The model under review builds one solid part; all positions refer to its coordinate system, in mm. Face numbers are marked on the shaded views. A direction names the side the tool comes from. Round coordinates to 2 decimals unless told otherwise and drop trailing zeros. Order: outer loops, then holes, each group sorted by start corner. A loop starts at its lowest first (then second) coordinate and runs counter-clockwise, first axis right, second up. Notation, with made-up numbers: M 27,17.25 L 32,17.25 A23 cw 32,38.25 Z; hole C 16,-17 d11. An arc over 180 degrees is marked long. One line per item, written item: value. Start each with the question number.
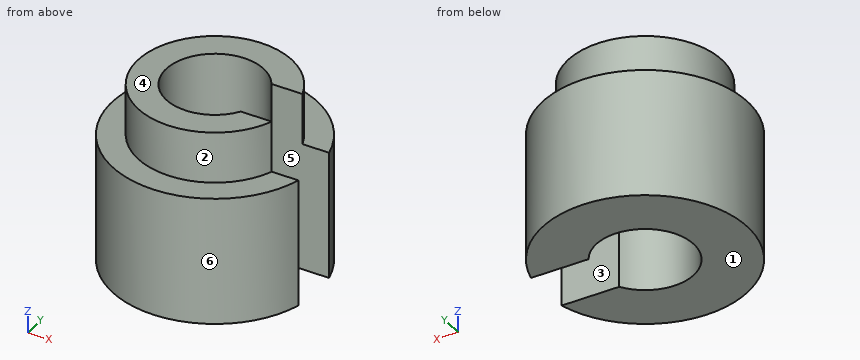
from build123d import *

# Parameters (mm, degrees)
SKETCH_1_R          = 4
EXTRUDE_1_DEPTH     = 5
SKETCH_2_R          = 3
EXTRUDE_2_DEPTH     = 2
SKETCH_3_R          = 1.9
CUT_EXTRUDE_1_DEPTH = 10
CUT_EXTRUDE_2_DEPTH = 1


with BuildPart() as part:
    # 草图1 → 凸台-拉伸1 (new body)
    with BuildSketch(Plane.XY):
        Circle(SKETCH_1_R)
    extrude(amount=EXTRUDE_1_DEPTH)

    # 草图2 → 凸台-拉伸2 (add)
    with BuildSketch(Plane.XY.offset(5)):
        Circle(SKETCH_2_R)
    extrude(amount=EXTRUDE_2_DEPTH)

    # 草图3 → 切除-拉伸1 (cut, through all)
    with BuildSketch(Plane.XY.offset(7)):
        Circle(SKETCH_3_R)
    extrude(amount=-CUT_EXTRUDE_1_DEPTH, mode=Mode.SUBTRACT)

    # 草图4 → 切除-拉伸2 (cut, symmetric)
    with BuildSketch(Plane(origin=(0, 0, 0), x_dir=(1, 0, 0), z_dir=(0, 1, 0))):
        Polygon((0, 0), (4, 0), (4, -5), (3, -5), (3, -7), (0, -7), align=None)
    extrude(amount=CUT_EXTRUDE_2_DEPTH, both=True, mode=Mode.SUBTRACT)


solid = part.part
Item 1: Consider section D-D, the plane z = 6. Give the boundary of the cut face in (x, y).
Item 2: Consider section B-B, the plane y = -1.5. Give the boundary of the cut face in (x, z).
Item 3: Machinability: for the marked faces 1, 2 and 3, which of the approach directions +Z, -Z, +X, -X, +Y, -Y give a long, thin tool a straight path to every point of the face, cutting with its end or side? Answer none if there is none.
Item 4: Consider section C-C, the plane y = 0. Give the boundary of the cut face in (x, z), then the cut area to 3 significant figures.
Item 5: Wall thickness on L1, parallel to Z at x = -1.75, y = -2.75; L2, parallel to Y at x = 2, z = 1.25; L3, parallel to X at y = 0, z = 2.75: over which ranges is each line inside the solid? List them lowest first.
Item 6: Consider section A-A, the plane x = 0. Give the boundary of the cut face in (y, z).
Item 7: The part is to be moulded in two halves that separate along Y. For the marked faces 4, 5 and 6, say which applies: pulls with the +Y half, pulls with the -Y half, needs draft (parallel to the pull), parting line crosses it, or undercut.
Item 8: Clearance check with flat-ended pins moving along their axes: P1, Ø1.5, axis at x = -2.5, z = 4, coming from the +Y side; P2, Ø0.7, axis at x = 2.5, z = 2.5, coming from the -Y side; P3, Ø1.1, axis at x = 3.5, z = 4.5, coming from the +Y side. State where each tip first meets the part, or that it passes through.
Computed:
1. outline: M 1.62,-1 A1.9 cw long 1.62,1 L 2.83,1 A3 ccw long 2.83,-1 Z
2. outline: M -3.71,0 L -1.17,0 L -1.17,7 L -2.6,7 L -2.6,5 L -3.71,5 Z; M 1.17,0 L 3.71,0 L 3.71,5 L 2.6,5 L 2.6,7 L 1.17,7 Z
3. face 1: -Z, +X, -X, +Y, -Y
3. face 2: +Z
3. face 3: +Z, -Z, +X
4. outline: M -4,0 L -1.9,0 L -1.9,7 L -3,7 L -3,5 L -4,5 Z
4. area: 12.7 mm^2
5. L1: z = 0 to 5
5. L2: y = -3.46 to -1, 1 to 3.46
5. L3: x = -4 to -1.9
6. outline: M -4,0 L -1.9,0 L -1.9,7 L -3,7 L -3,5 L -4,5 Z; M 1.9,0 L 4,0 L 4,5 L 3,5 L 3,7 L 1.9,7 Z
7. face 4: needs draft
7. face 5: undercut
7. face 6: parting line crosses it
8. P1: stops at y = 3.6
8. P2: stops at y = -3.37
8. P3: stops at y = 2.7
